from build123d import *

# Parameters (mm, degrees)
SKETCH1_R           = 9
BOSS_EXTRUDE1_DEPTH = 9
SKETCH2_R           = 5.5
CUT_EXTRUDE1_DEPTH  = 8
SKETCH3_R           = 1
CUT_EXTRUDE2_DEPTH  = 3


with BuildPart() as part:
    # Sketch1 → Boss-Extrude1 (new body)
    with BuildSketch(Plane(origin=(0, 0, 0), x_dir=(1, 0, 0), z_dir=(0, 1, 0))):
        Circle(SKETCH1_R)
    extrude(amount=BOSS_EXTRUDE1_DEPTH)

    # Sketch2 → Cut-Extrude1 (cut)
    with BuildSketch(Plane(origin=(0, 9, 0), x_dir=(1, 0, 0), z_dir=(0, 1, 0))):
        Circle(SKETCH2_R)
    extrude(amount=-CUT_EXTRUDE1_DEPTH, mode=Mode.SUBTRACT)

    # Sketch3 → Cut-Extrude2 (cut)
    with BuildSketch(Plane(origin=(0, 9, 0), x_dir=(1, 0, 0), z_dir=(0, 1, 0))):
        with Locations((0, 7.25)):
            Circle(SKETCH3_R)
        with Locations((0, -7.25)):
            Circle(SKETCH3_R)
    extrude(amount=-CUT_EXTRUDE2_DEPTH, mode=Mode.SUBTRACT)


solid = part.part
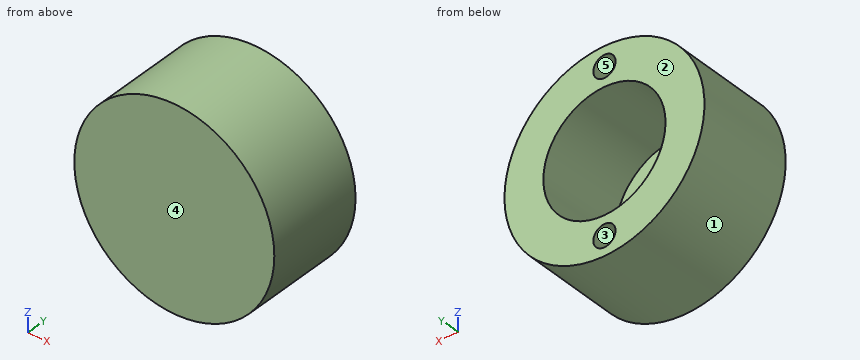
Work out the finished part from the listing and answer in its coordinate system (mm). Face numbers are marked on the shaded views. A direction names the side the tool comes from. Coordinates: 2 decimals unless noted, no trailing zeros. Write each loop counter-clockwise with the first axis right and the second up, starting at its lowest first coordinate (ties: lowest second). Pieces come first, ordered by that corner, then holes.
1. The part is cut by section A-A, the plane z = 0. Write down the section's boundary in (x, y).
Results list:
outline: (-9, 0) - (9, 0) - (9, 9) - (5.5, 9) - (5.5, 1) - (-5.5, 1) - (-5.5, 9) - (-9, 9) - close
2. For a pull along Z with two mould halves and no side action, classify the marked faces 1, 2 and 3 as +Z half, -Z half, draft (parallel to the pull), parting line (faces both ways), or undercut.
Results list:
face 1: parting line
face 2: draft
face 3: undercut
3. The part is cut by section D-D, the plane y = 6.5. Write down the section's boundary in (x, z).
Results list:
outline: circle Ø18 at (0, 0); hole circle Ø11 at (0, 0); hole circle Ø2 at (0, -7.25); hole circle Ø2 at (0, 7.25)
4. The part is cut by section C-C, the plane y = 4. Write down the section's boundary in (x, z), and give its area (3 significant figures).
Results list:
outline: circle Ø18 at (0, 0); hole circle Ø11 at (0, 0)
area: 159 mm2
5. Consider line 1 along X through (y, z) = (5.75, 0); line 2 along Z through (x, y) = (-0.5, 5.5); line 3 along X through (y, z) = (4, -3.5). Determine where each line is inside the solid, lowest interval first.
Results list:
line 1: x = -9 to -5.5, 5.5 to 9
line 2: z = -8.99 to -5.48, 5.48 to 8.99
line 3: x = -8.29 to -4.24, 4.24 to 8.29
6. Flat-ended cylindrical pins translate along their axes: pin 1 (5 mm diameter, centred on x = 7, y = 1, fed in from +Z); pin 2 (1.6 mm diameter, centred on x = 0, z = 7.25, fed in from +Y); pin 3 (1.5 mm diameter, centred on x = 3, z = 1.5, fed in from +Y). Find the tip coordinate at first contact, or state that the pin passes through.
Results list:
pin 1: stops at z = 7.79
pin 2: stops at y = 6
pin 3: stops at y = 1
7. The part is cut by section B-B, the plane x = 0. Write down the section's boundary in (y, z).
Results list:
outline: (0, -9) - (9, -9) - (9, -8.25) - (6, -8.25) - (6, -6.25) - (9, -6.25) - (9, -5.5) - (1, -5.5) - (1, 5.5) - (9, 5.5) - (9, 6.25) - (6, 6.25) - (6, 8.25) - (9, 8.25) - (9, 9) - (0, 9) - close
8. For the marked faces 4 and 5, determine the directions among +Z, -Z, +X, -X, +Y, -Y from which every point of the face is accessible in a straight line to the end or side of a thin tool.
Results list:
face 4: +Z, -Z, +X, -X, -Y
face 5: +Y
